Check sheet for the modelled part. Datum: model origin and axes. Units: mm. Face numbers are marked on the shaded views. A direction names the side the tool comes from. Round coordinates to 2 decimals unless told otherwise and drop trailing zeros. Order: outer loops, then holes, each group sorted by start corner. A loop starts at its lowest first (then second) coordinate and runs counter-clockwise, first axis right, second up. Notation, with made-up numbers: M 24,13.5 L 45,13.5 A16 cw 45,26.5 Z; hole C -18,32.5 d2. An arc over 180 degrees is marked long. One line per item, written item: value. Start each with the question number.
(1) Cross-section at A-A, the plane x = -12.7. Enter the section's corners in (y, z), and give its area (3 significant figures).
(2) Depth check by flat-ended pin: pin 1 Ø4 at (x, z) = (-45.5, 4) entering from -Y; pin 2 Ø1 at (y, z) = (-23.5, 3.5) entering from +X; pin 3 Ø10 at (y, z) = (-13, 12) entering from +X. Enter the tip coordinate at first touch or a pass-through.
(3) Thickness scan on L1, parallel to Z at x = -35.5, y = -3.5; L2, parallel to X at y = -15, z = 10.5; L3, parallel to X at y = -22.5, z = 13.75. Record the ranges inside material, lowest first.
(4) Access from +Z, -Z, +X, -X, +Y, -Y to the whole of each face (thin tool, end or side, straight path). Record for the marked faces 1 and 2.
(5) Cross-section at C-C, the plane z = 6.75. Enter the section's corners in (x, y), and give its area (3 significant figures).
(6) Cross-section at D-D, the plane y = -23. Enter the section's corners in (x, z), and give its area (3 significant figures).
(7) Cross-section at B-B, the plane y = -15.24. Enter the section's corners in (x, z), and give its area (3 significant figures).
from build123d import *

# Parameters (mm, degrees)
F0_W     = 127
F0_H     = 50.8
F1_DEPTH = 0.508
F3_DEPTH = 12.7
F5_DEPTH = 5.08


with BuildPart() as f1:
    # F0 (on Top) → F1 (new body)
    with BuildSketch(Plane.XY):
        with Locations((-63.5, -25.4)):
            Rectangle(F0_W, F0_H)
    extrude(amount=F1_DEPTH)

    # F2 (on face) → F3 (join)
    with BuildSketch(Plane.XY.offset(0.508)):
        with BuildLine():
            ThreePointArc((-20.399375, -19.6842912381), (-10.3994939415, -23.8271864935), (-3.81, -15.24))
            ThreePointArc((-3.81, -15.24), (-10.3994939415, -6.6528135065), (-20.399375, -10.7957087619))
            ThreePointArc((-20.399375, -10.7957087619), (-18.4835645212, -12.6606178065), (-17.78, -15.24))
            ThreePointArc((-17.78, -15.24), (-18.4835645212, -17.8193821935), (-20.399375, -19.6842912381))
        make_face()
        with BuildLine():
            ThreePointArc((-17.78, -15.24), (-18.4835645212, -12.6606178065), (-20.399375, -10.7957087619))
            ThreePointArc((-20.399375, -10.7957087619), (-21.59, -15.24), (-20.399375, -19.6842912381))
            ThreePointArc((-20.399375, -19.6842912381), (-18.4835645212, -17.8193821935), (-17.78, -15.24))
        make_face()
        with BuildLine():
            ThreePointArc((-20.399375, -19.6842912381), (-21.59, -15.24), (-20.399375, -10.7957087619))
            ThreePointArc((-20.399375, -10.7957087619), (-27.94, -15.24), (-20.399375, -19.6842912381))
        make_face()
    extrude(amount=F3_DEPTH)

    # F4 (on face) → F5 (join)
    with BuildSketch(Plane.XY.offset(13.208)):
        with BuildLine():
            ThreePointArc((-20.399375, -19.6842912381), (-10.3994939415, -23.8271864935), (-3.81, -15.24))
            ThreePointArc((-3.81, -15.24), (-10.3994939415, -6.6528135065), (-20.399375, -10.7957087619))
            ThreePointArc((-20.399375, -10.7957087619), (-21.59, -15.24), (-20.399375, -19.6842912381))
        make_face()
    extrude(amount=F5_DEPTH)


solid = f1.part
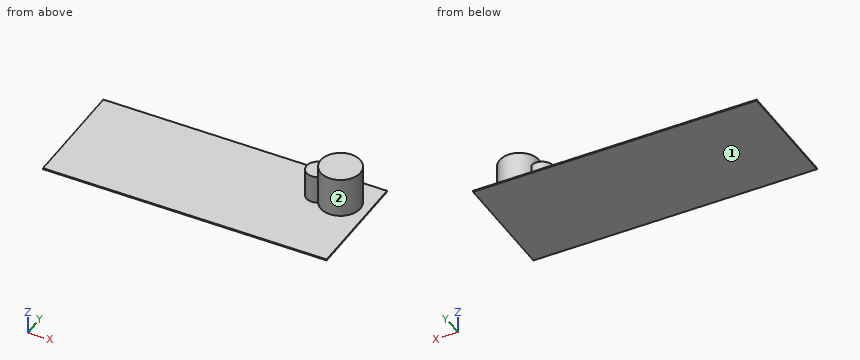
Values found:
1. outline: M -50.8,0 L 0,0 L 0,0.51 L -6.35,0.51 L -6.35,18.29 L -24.13,18.29 L -24.13,0.51 L -50.8,0.51 Z
1. area: 342 mm^2
2. pin 1: through
2. pin 2: x = -8.36
2. pin 3: x = -3.81
3. L1: 0 to 0.51
3. L2: -27.93 to -3.81
3. L3: -17.83 to -7.57
4. face 1: -Z, +X, -X, +Y, -Y
4. face 2: +Z
5. outline: M -20.4,-19.68 A8.89 ccw long -20.4,-10.8 A5.08 ccw long Z
5. area: 306 mm^2
6. outline: M -127,0 L 0,0 L 0,0.51 L -8.36,0.51 L -8.36,18.29 L -17.04,18.29 L -17.04,0.51 L -127,0.51 Z
6. area: 219 mm^2
7. outline: M -127,0 L 0,0 L 0,0.51 L -3.81,0.51 L -3.81,18.29 L -21.59,18.29 L -21.59,13.21 L -27.94,13.21 L -27.94,0.51 L -127,0.51 Z
7. area: 461 mm^2
